Check sheet for the modelled part. Datum: model origin and axes. Units: mm. Face numbers are marked on the shaded views. A direction names the side the tool comes from. Round coordinates to 2 decimals unless told otherwise and drop trailing zeros. Loops run counter-clockwise (first coordinate to the right, second up) from the corner with the lowest first, then second, coordinate; pieces in that order, holes last. Notation, with made-up numbers: (-6, 15.5) - (36, 15.5) arc R28 cw to (36, 49.5) - close; hole circle Ø3 at (73, 29). An arc over 180 degrees is marked (long way). Answer in a Markdown table with one row per item. Add a question column.
(1) Cross-section at B-B on x = 10.5. Enter the section's corners in (y, z).
(2) Cross-section at C-C on z = 15. Enter the section's corners in (x, y), then the cut area to 3 significant figures.
(3) Thickness scan on line 1 along X through (y, z) = (-19, 16); line 2 along Y through (x, z) = (-3, 6.5); line 3 along X through (y, z) = (-15.5, 1.5). Record the ranges inside material, lowest first.
(4) Gauge pin test, flat ends, axial feed: pin 1 (1 mm diameter, centred on y = -34, z = -5.5, fed in from +X); pin 2 (11.5 mm diameter, centred on x = -25.5, y = -42.5, fed in from -Z); pin 3 (1.5 mm diameter, centred on x = -47, y = -54, fed in from +Z); pin 4 (17.5 mm diameter, centred on x = 34.21, z = 9.98, fed in from -Y). Record the tip position at first contact, or that the pin passes through.
(5) Mould release check, pull along Z, two halves, no side actions. Record for the marked faces 1, 2, 3 and 4: +Z half, -Z half, draft (parallel to the pull), parting line (faces both ways), or undercut.
(6) Cross-section at A-A on z = -2.5. Enter the section's corners in (x, y), then the cut area to 3 significant figures.
(7) Access from +Z, -Z, +X, -X, +Y, -Y to the whole of each face (thin tool, end or side, straight path). Record for the marked faces 5, 6, 7 and 8.
(8) Cross-section at D-D on y = -58.5. Enter the section's corners in (x, z).
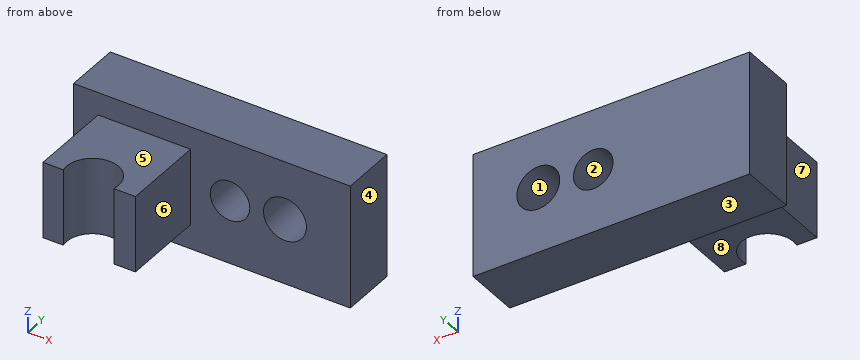
from build123d import *

# Parameters (mm, degrees)
F0_W     = 125.667088
F0_H     = 56.080402
F1_DEPTH = 25.4
F2_W     = 41.9869
F2_H     = 34.646532
F3_DEPTH = 38.1
F5_DEPTH = 50.8
F6_R     = 8.98768
F6_R_2   = 9.7602
F7_DEPTH = 50.8


with BuildPart() as f1:
    # F0 (on Front) → F1 (new body)
    with BuildSketch(Plane.XZ):
        with Locations((1.027655, 8.368018)):
            Rectangle(F0_W, F0_H)
    extrude(amount=F1_DEPTH)

    # F2 (on face) → F3 (join)
    with BuildSketch(Plane.XZ.offset(25.4)):
        with Locations((-29.655083, 8.80844)):
            Rectangle(F2_W, F2_H)
    extrude(amount=F3_DEPTH)

    # F4 (on face) → F5 (cut)
    with BuildSketch(Plane(origin=(0, 0, -8.514826), x_dir=(1, 0, 0), z_dir=(0, 0, -1))):
        with BuildLine():
            Line((-18.516481, 63.5), (-41.419674, 63.5))
            ThreePointArc((-41.419674, 63.5), (-29.968077, 49.006404), (-18.516481, 63.5))
        make_face()
    extrude(amount=-F5_DEPTH, mode=Mode.SUBTRACT)

    # F6 (on face) → F7 (cut)
    with BuildSketch(Plane.XZ.offset(25.4)):
        with Locations((9.248862, 9.102055)):
            Circle(F6_R)
        with Locations((34.206115, 9.982899)):
            Circle(F6_R_2)
    extrude(amount=-F7_DEPTH, mode=Mode.SUBTRACT)


solid = f1.part
Answers:
| question | item | result |
|---|---|---|
| 1 | outline | (-25.4, -19.67) - (0, -19.67) - (0, 0.2) - (-25.4, 0.2) - close; (-25.4, 18) - (0, 18) - (0, 36.41) - (-25.4, 36.41) - close |
| 2 | outline | (-61.81, -25.4) - (-50.65, -25.4) - (-50.65, -63.5) - (-41.42, -63.5) arc R11.77 cw (long way) to (-18.52, -63.5) - (-8.66, -63.5) - (-8.66, -25.4) - (2.47, -25.4) - (2.47, 0) - (-61.81, 0) - close; (16.03, -25.4) - (25.83, -25.4) - (25.83, 0) - (16.03, 0) - close; (42.58, -25.4) - (63.86, -25.4) - (63.86, 0) - (42.58, 0) - close |
| 2 | area | 3,740 mm^2 |
| 3 | line 1 | x = -61.81 to 3.49, 15.01 to 26.52, 41.89 to 63.86 |
| 3 | line 2 | y = -25.4 to 0 |
| 3 | line 3 | x = -61.81 to 4.45, 14.04 to 29.38, 39.03 to 63.86 |
| 4 | pin 1 | stops at x = -8.66 |
| 4 | pin 2 | stops at z = -8.51 |
| 4 | pin 3 | stops at z = 26.13 |
| 4 | pin 4 | passes through |
| 5 | face 1 | undercut |
| 5 | face 2 | undercut |
| 5 | face 3 | -Z half |
| 5 | face 4 | draft |
| 6 | outline | (-61.81, -25.4) - (-50.65, -25.4) - (-50.65, -63.5) - (-41.42, -63.5) arc R11.77 cw (long way) to (-18.52, -63.5) - (-8.66, -63.5) - (-8.66, -25.4) - (63.86, -25.4) - (63.86, 0) - (-61.81, 0) - close |
| 6 | area | 4,510 mm^2 |
| 7 | face 5 | +Z, +X, -X, -Y |
| 7 | face 6 | +Z, -Z, +X, -Y |
| 7 | face 7 | +Z, -Z, -X, -Y |
| 7 | face 8 | -Z, +X, -X, -Y |
| 8 | outline | (-50.65, -8.51) - (-41.52, -8.51) - (-41.52, 26.13) - (-50.65, 26.13) - close; (-18.42, -8.51) - (-8.66, -8.51) - (-8.66, 26.13) - (-18.42, 26.13) - close |
